Build history of the part. All positions in model axes, mm. A direction names the side the tool comes from. Give positions to 0.01 mm unless a question says otherwise; leave off trailing zeros. Loops run counter-clockwise (first coordinate to the right, second up) from the corner with the lowest first, then second, coordinate; pieces in that order, holes last. Notation, with made-up numbers: M -34.5,81 L -2.5,81 A17 cw -2.5,110 Z; hole C -27,30 d7. An arc over 180 degrees is marked long. Answer as a JSON object with one key per item and string values. Group by question number.
1. Slice it at C-C (x = 29.5). List the corners of the cut face in (y, z), then the cut area to 3 significant figures.
2. Mould opens along X. For faces 1 (the face through (24.843, 50.287, -1.259)), 2 (the face through (50.287, 50.259, 8.112)), 3 (the face through (45.74, 43.58, -0.89)) say: released by +X, released by -X, zero draft, split by the parting line, or undercut.
3. Slice it at D-D (y = 35). List the corners of the cut face in (x, z), then the cut area to 3 significant figures.
4. 3-axis set-ups, long thin cutter, end or side, ignore diameter. For faces 4 (the face through (28, -1, 5.5)), 5 (the face through (0, 24, 8)), 6 (the face through (-1, 36, 11)): which of +Z, -Z, +X, -X, +Y, -Y reach the whole face in a straight line?
5. Slice it at B-B (y = 4). List the corners of the cut face in (x, z).
6. Drop flat-ended pins along their axis: pin 1 Ø12 at (x, y) = (34, 30) entering from +Z; pin 2 Ø2 at (x, y) = (32.5, -1.5) entering from -Z; pin 3 Ø0.9 at (x, z) = (-1.5, 8) entering from -Y. Give the stop position or say it passes through.
7. Slice it at A-A (z = 8.5). List the corners of the cut face in (x, y).
8. Drill centre lines: line 1 along Y through (x, z) = (18, 4.25); line 2 along Y through (x, z) = (45, -0.4) (3 decimals). Where is each one in solid material? Low to high. Write a range as [from, to].
from build123d import *

# Parameters (mm, degrees)
SKETCH_W        = 49
SKETCH_H        = 49
PAD_DEPTH       = 16
THICKNESS_T     = 1.8
SKETCH001_R     = 1.6
POCKET_DEPTH    = 1.801
SKETCH002_W     = 29
SKETCH002_H     = 7
POCKET001_DEPTH = 1.8
SKETCH003_W     = 11
SKETCH003_H     = 5.5
POCKET002_DEPTH = 1.8


with BuildPart() as part:
    # Sketch → Pad (new body)
    with BuildSketch(Plane.XY):
        with Locations((24.5, 24.5)):
            Rectangle(SKETCH_W, SKETCH_H)
    extrude(amount=PAD_DEPTH)

    # Thickness
    thickness_openings = [part.faces().sort_by_distance(p)[0] for p in [
        (24.5, 24.5, 16),
    ]]
    offset(amount=THICKNESS_T, openings=thickness_openings)

    # Sketch001 → Pocket (cut, through all)
    with BuildSketch(Plane.XY):
        with Locations((4, 45)):
            Circle(SKETCH001_R)
        with Locations((4, 4)):
            Circle(SKETCH001_R)
        with Locations((45, 45)):
            Circle(SKETCH001_R)
        with Locations((45, 4)):
            Circle(SKETCH001_R)
    extrude(amount=-POCKET_DEPTH, mode=Mode.SUBTRACT)

    # Sketch002 → Pocket001 (cut)
    with BuildSketch(Plane.XZ.offset(1.8)):
        with Locations((28.5, 9)):
            Rectangle(SKETCH002_W, SKETCH002_H)
    extrude(amount=-POCKET001_DEPTH, mode=Mode.SUBTRACT)

    # Sketch003 → Pocket002 (cut)
    with BuildSketch(Plane(origin=(-1.8, 0, 0), x_dir=(0, -1, 0), z_dir=(-1, 0, 0))):
        with Locations((-35.5, 8.25)):
            Rectangle(SKETCH003_W, SKETCH003_H)
    extrude(amount=-POCKET002_DEPTH, mode=Mode.SUBTRACT)


solid = part.part
Established:
{
 "1": {"outline": "M -1.8,0 A1.8 ccw 0,-1.8 L 49,-1.8 A1.8 ccw 50.8,0 L 50.8,16 L 49,16 L 49,0 L 0,0 L 0,5.5 L -1.8,5.5 Z; M -1.8,12.5 L 0,12.5 L 0,16 L -1.8,16 Z", "area": "138 mm^2"},
 "2": {"face 1": "zero draft", "face 2": "released by +X", "face 3": "undercut"},
 "3": {"outline": "M -1.8,0 A1.8 ccw 0,-1.8 L 49,-1.8 A1.8 ccw 50.8,0 L 50.8,16 L 49,16 L 49,0 L 0,0 L 0,5.5 L -1.8,5.5 Z; M -1.8,11 L 0,11 L 0,16 L -1.8,16 Z", "area": "141 mm^2"},
 "4": {"face 4": "-Y", "face 5": "+Z", "face 6": "-X"},
 "5": {"outline": "M -1.8,0 A1.8 ccw 0,-1.8 L 2.4,-1.8 L 2.4,0 L 0,0 L 0,16 L -1.8,16 Z; M 5.6,-1.8 L 43.4,-1.8 L 43.4,0 L 5.6,0 Z; M 46.6,-1.8 L 49,-1.8 A1.8 ccw 50.8,0 L 50.8,16 L 49,16 L 49,0 L 46.6,0 Z"},
 "6": {"pin 1": "stops at z = 0", "pin 2": "stops at z = -1.73", "pin 3": "stops at y = -1.46"},
 "7": {"outline": "M -1.8,0 A1.8 ccw 0,-1.8 L 14,-1.8 L 14,0 L 0,0 L 0,30 L -1.8,30 Z; M -1.8,41 L 0,41 L 0,49 L 49,49 L 49,0 L 43,0 L 43,-1.8 L 49,-1.8 A1.8 ccw 50.8,0 L 50.8,49 A1.8 ccw 49,50.8 L 0,50.8 A1.8 ccw -1.8,49 Z"},
 "8": {"line 1": "y = [-1.8, 0], [49, 50.8]", "line 2": "y = [-1.755, 2.4], [5.6, 43.4], [46.6, 50.755]"}
}
